CAD build for the part. Positions are in the model's coordinates, mm. A direction names the side the tool comes from. Coordinates: 2 decimals unless noted, no trailing zeros. Loops run counter-clockwise (first coordinate to the right, second up) from the corner with the lowest first, then second, coordinate; pieces in that order, holes last. Notation, with made-up numbers: (16.25, 34) -> (59.25, 34) arc R25 ccw to (59.25, 49) -> close; hole circle Ø2 at (-34.75, 36). An arc over 180 degrees is marked (long way). Write item = value, one per line. Start each with the question number.
(1) Band-saw the part on D-D (y = -28.5). Write the cut outline in (x, z), and give its area (3 significant figures).
(2) Band-saw the part on B-B (y = -12.5). Write the cut outline in (x, z), and give its area (3 significant figures).
(3) Band-saw the part on C-C (z = 0). Write the cut outline in (x, y), and give its area (3 significant figures).
(4) Pull direction X, two halves, no side cores. Call faces 3 (the face through (-7.294, -25.044, 55.555)), 4 (the face through (-34, 0, 52)), 5 (the face through (76.757, -13, -1)): +X half, -X half, draft (parallel to the pull), parting line (faces both ways), or undercut.
(5) Tool access for faces 1 (the face through (33.54, -37.92, 52.6)), 2 (the face through (-1, -13, 76.034)): list every direction of +Z, -Z, +X, -X, +Y, -Y with a clear straight run to the whole face (end or side of a thin tool).
(6) Flat gauge pins, fed straight in: P1, Ø6, axis at y = -41.5, z = 8.5, coming from the -X side; P2, Ø1, axis at y = -31, z = -46.5, coming from the -X side; P3, Ø8, axis at x = 20, y = -37.5, coming from the -Z side. Where does each tip first touch, or does it go through?
(7) Drill centre lines: line 1 (Z direction, x = 0, y = -13.5); line 2 (Z direction, x = 0, y = -35.5); line 3 (Y direction, x = 19.5, z = 66). Where is each one in solid material? Low to high. Write a range as from..to.
(8) Band-saw the part on A-A (x = 0). Write the cut outline in (y, z).
```python
from build123d import *

# Parameters (mm, degrees)
F0_W     = 152.549193
F0_H     = 152.0672
F0_R     = 62.382267
F1_DEPTH = 25.4
F0_R_2   = 56.032267
F2_DEPTH = 50.8


with BuildPart() as f1:
    # F0 (on Front) → F1 (new body)
    with BuildSketch(Plane.XZ):
        with Locations((0.481986, 0)):
            Rectangle(F0_W, F0_H)
        Circle(F0_R, mode=Mode.SUBTRACT)
    extrude(amount=F1_DEPTH)

    # F0 (on Front) → F2 (join)
    with BuildSketch(Plane.XZ):
        Circle(F0_R)
        Circle(F0_R_2, mode=Mode.SUBTRACT)
    extrude(amount=F2_DEPTH)


solid = f1.part
```
Findings below:
q1.outline = circle Ø124.76 at (0, 0); hole circle Ø112.06 at (0, 0)
q1.area = 2,360 mm²
q2.outline = (-75.79, -76.03) -> (76.76, -76.03) -> (76.76, 76.03) -> (-75.79, 76.03) -> close; hole circle Ø112.06 at (0, 0)
q2.area = 13,300 mm²
q3.outline = (-75.79, -25.4) -> (-62.38, -25.4) -> (-62.38, -50.8) -> (-56.03, -50.8) -> (-56.03, 0) -> (-75.79, 0) -> close; (56.03, -50.8) -> (62.38, -50.8) -> (62.38, -25.4) -> (76.76, -25.4) -> (76.76, 0) -> (56.03, 0) -> close
q3.area = 1,350 mm²
q4.face_3 = undercut
q4.face_4 = draft
q4.face_5 = +X half
q5.face_1 = -Y
q5.face_2 = +Z, +X, -X, +Y, -Y
q6.P1 = -62.14
q6.P2 = -42.14
q6.P3 = -60.3
q7.line_1 = -76.03..-56.03, 56.03..76.03
q7.line_2 = -62.38..-56.03, 56.03..62.38
q7.line_3 = -25.4..0
q8.outline = (-50.8, -62.38) -> (-25.4, -62.38) -> (-25.4, -76.03) -> (0, -76.03) -> (0, -56.03) -> (-50.8, -56.03) -> close; (-50.8, 56.03) -> (0, 56.03) -> (0, 76.03) -> (-25.4, 76.03) -> (-25.4, 62.38) -> (-50.8, 62.38) -> close
